Source: three-view drawing plus pictorial views. Frame: mm from the lowest corner of the part. Round coordinates to 2 decimals unless told otherwise and drop trailing zeros. Loops run counter-clockwise (first coordinate to the right, second up) from the corner with the lowest first, then second, coordinate; pieces in that order, holes last. Notation, with made-up numbers: (5, -21.5) -> (11, -21.5) arc R20 cw to (11, 10.5) -> close; hole circle Ø9 at (46.25, -34.75). An arc over 180 degrees is marked (long way). Answer as a JSON object with one key per item and string values. Group by question number.
Item 1: Material intervals for line 1 (Y direction, x = 0.75, z = 8); line 2 (Z direction, x = 0.2, y = 2); line 3 (Y direction, x = 1.3, z = 44), sorted ascending. Write a range as [from, to].
Item 2: Pin query (flat end, axial travel): pin 1 (1 mm diameter, centred on x = 0.5, z = 5, fed in from -Y). Return the tip coordinate at first contact, or that it passes through.
Item 3: Section query A-A on y = 4. Return loops of the section in (x, z).
Item 4: Section query C-C on z = 116.5. Return loops of the section in (x, y), and give its area (3 significant figures).
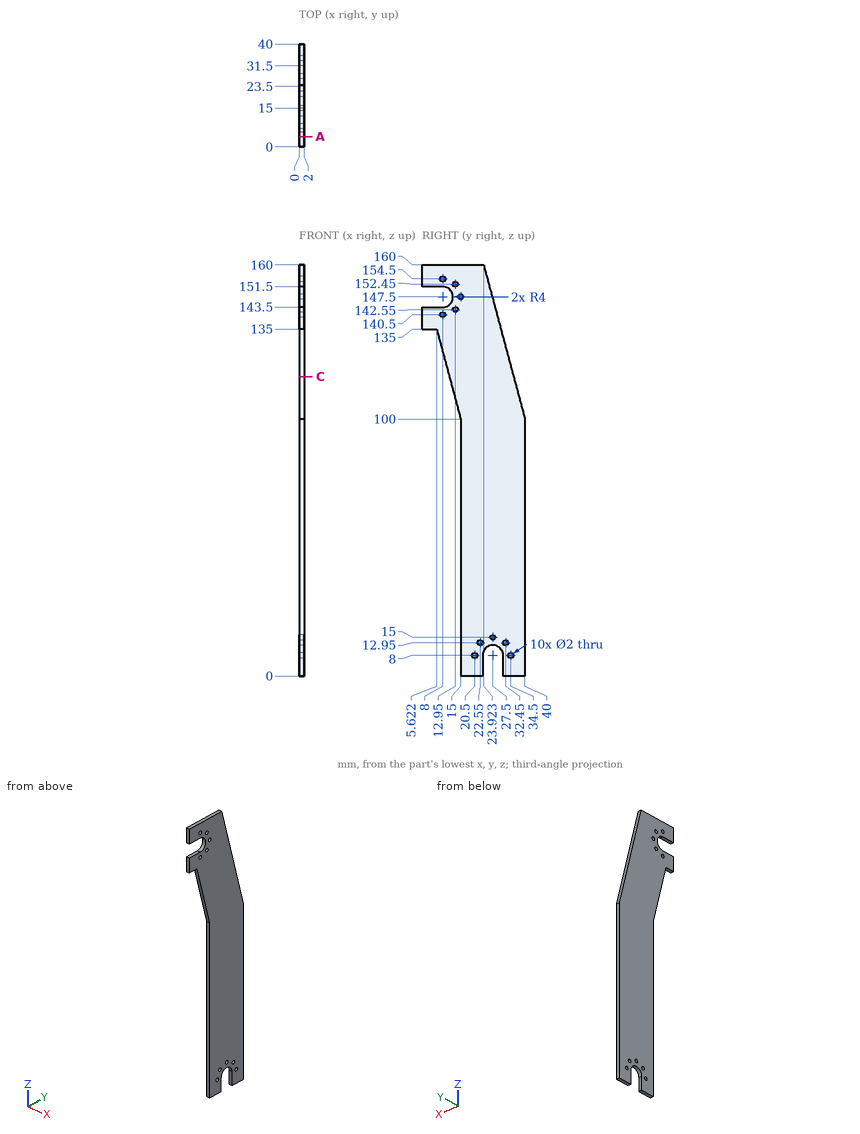
Solved:
{
 "1": {"line 1": "[15, 19.5], [21.5, 23.5], [31.5, 33.5], [35.5, 40]", "line 2": "[135, 143.5], [151.5, 160]", "line 3": "[15, 40]"},
 "2": {"pin 1": "y = 15"},
 "3": {"outline": "(0, 135) -> (2, 135) -> (2, 143.5) -> (0, 143.5) -> close; (0, 151.5) -> (2, 151.5) -> (2, 160) -> (0, 160) -> close"},
 "4": {"outline": "(0, 10.58) -> (2, 10.58) -> (2, 35.58) -> (0, 35.58) -> close", "area": "50.0 mm²"}
}
